Design review of the part built by this model. Coordinates are the model's own, in mm. A direction names the side the tool comes from. Give positions to 0.01 mm unless a question says otherwise; leave off trailing zeros. Order: outer loops, then holes, each group sorted by start corner. A loop starts at its lowest first (then second) coordinate and runs counter-clockwise, first axis right, second up. Notation, with made-up numbers: (47.5, -34) -> (104.5, -34) arc R27 cw to (104.5, -13) -> close; hole circle Ø2 at (-26.75, 45). An arc over 180 degrees is marked (long way). Return JSON: item names as keys, results as strings.
```python
from build123d import *

# Parameters (mm, degrees)
SKETCH_1_W               = 20
SKETCH_1_H               = 200
SKETCH_1_W_2             = 80
EXTRUDE_1_DEPTH          = 3
SKETCH_3_W               = 200
SKETCH_3_H               = 3
REVOLVE_1_ANGLE          = 90
SKETCH_5_W               = 200
SKETCH_5_H               = 3
REVOLVE_2_ANGLE          = 90
SKETCH_7_R               = 28.5
EXTRUDE_4_DEPTH          = 55
SKETCH_7_6_R             = 28.5
CUT_EXTRUDE_1_DEPTH      = 47
SKETCH_9_R               = 1.65
CUT_EXTRUDE_2_DEPTH      = 47
SKETCH_10_R              = 1.65
CUT_EXTRUDE_3_DEPTH      = 47
EXTRUDE_5_DEPTH          = 55
SKETCH_11_3_R            = 28.5
CUT_EXTRUDE_4_DEPTH      = 47
SKETCH_14_R              = 1.65
CUT_EXTRUDE_5_DEPTH      = 47
SKETCH_15_W              = 60
SKETCH_15_H              = 86
EXTRUDE_6_DEPTH          = 3
SKETCH_17_W              = 5
SKETCH_17_H              = 10
SKETCH_17_R              = 1.65
EXTRUDE_7_DEPTH          = 5
SKETCH_18_W              = 5
SKETCH_18_H              = 10
SKETCH_18_R              = 1.65
EXTRUDE_8_DEPTH          = 5
CUT_EXTRUDE_6_DEPTH      = 11
SKETCH_20_W              = 5.5
SKETCH_20_H              = 8.5
CUT_EXTRUDE_7_DEPTH      = 108
CUT_EXTRUDE_7_DEPTH_BACK = 119


with BuildPart() as part:
    # Sketch 1 → Extrude 1 (new body)
    with BuildSketch(Plane(origin=(0, 0, 0), x_dir=(1, 0, 0), z_dir=(0, 1, 0))):
        with Locations((-50, 0)):
            Rectangle(SKETCH_1_W, SKETCH_1_H)
        Rectangle(SKETCH_1_W_2, SKETCH_1_H)
        with Locations((50, 0)):
            Rectangle(SKETCH_1_W, SKETCH_1_H)
    extrude(amount=EXTRUDE_1_DEPTH)

    # Sketch 3 → Revolve 1 (revolve)
    with BuildSketch(Plane(origin=(60, 0, 0), x_dir=(0, 0, -1), z_dir=(1, 0, 0))):
        with Locations((0, 1.5)):
            Rectangle(SKETCH_3_W, SKETCH_3_H)
    revolve(axis=Axis((60, 33, 100), (0, 0, 1)), revolution_arc=REVOLVE_1_ANGLE)

    # Sketch 5 → Revolve 2 (revolve)
    with BuildSketch(Plane.ZY.offset(60)):
        with Locations((0, 1.5)):
            Rectangle(SKETCH_5_W, SKETCH_5_H)
    revolve(axis=Axis((-60, 33, -100), (0, 0, -1)), revolution_arc=REVOLVE_2_ANGLE)

    # Sketch 7 → Extrude 4 (add)
    with BuildSketch(Plane.XY.offset(100)):
        with Locations((-40, 40)):
            Circle(SKETCH_7_R)
        with BuildLine():
            Line((-60, 3), (-20, 3))
            Line((-20, 3), (-20, 19.696059496))
            ThreePointArc((-20, 19.696059496), (-40, 11.5), (-60, 19.696059496))
            Line((-60, 19.696059496), (-60, 3))
        make_face()
        with Locations((40, 40)):
            Circle(SKETCH_7_R)
        with BuildLine():
            Line((60, 3), (60, 19.696059496))
            ThreePointArc((60, 19.696059496), (40, 11.5), (20, 19.696059496))
            Line((20, 19.696059496), (20, 3))
            Line((20, 3), (60, 3))
        make_face()
    extrude(amount=-EXTRUDE_4_DEPTH)

    # Sketch 7_6 → Cut-Extrude 1 (cut)
    with BuildSketch(Plane.XY.offset(100)):
        with Locations((40, 40)):
            Circle(SKETCH_7_6_R)
        with Locations((-40, 40)):
            Circle(SKETCH_7_6_R)
    extrude(amount=-CUT_EXTRUDE_1_DEPTH, mode=Mode.SUBTRACT)

    # Sketch 9 → Cut-Extrude 2 (cut)
    with BuildSketch(Plane(origin=(0, 0, 45), x_dir=(-1, 0, 0), z_dir=(0, 0, -1))):
        with Locations((-53.435028843, 53.435028843)):
            Circle(SKETCH_9_R)
        with Locations((-26.564971157, 53.435028843)):
            Circle(SKETCH_9_R)
        with Locations((-26.564971157, 26.564971157)):
            Circle(SKETCH_9_R)
        with Locations((-53.435028843, 26.564971157)):
            Circle(SKETCH_9_R)
    extrude(amount=-CUT_EXTRUDE_2_DEPTH, mode=Mode.SUBTRACT)

    # Sketch 10 → Cut-Extrude 3 (cut)
    with BuildSketch(Plane(origin=(0, 0, 45), x_dir=(-1, 0, 0), z_dir=(0, 0, -1))):
        with Locations((26.564971157, 53.435028843)):
            Circle(SKETCH_10_R)
        with Locations((53.435028843, 53.435028843)):
            Circle(SKETCH_10_R)
        with Locations((53.435028843, 26.564971157)):
            Circle(SKETCH_10_R)
        with Locations((26.564971157, 26.564971157)):
            Circle(SKETCH_10_R)
    extrude(amount=-CUT_EXTRUDE_3_DEPTH, mode=Mode.SUBTRACT)

    # Sketch 11 → Extrude 5 (add)
    with BuildSketch(Plane(origin=(0, 0, -100), x_dir=(-1, 0, 0), z_dir=(0, 0, -1))):
        with BuildLine():
            Line((-20, 3), (-20, 19.696059496))
            ThreePointArc((-20, 19.696059496), (-40, 68.5), (-60, 19.696059496))
            Line((-60, 19.696059496), (-60, 3))
            Line((-60, 3), (-20, 3))
        make_face()
        with BuildLine():
            Line((20, 19.696059496), (20, 3))
            Line((20, 3), (60, 3))
            Line((60, 3), (60, 19.696059496))
            ThreePointArc((60, 19.696059496), (40, 68.5), (20, 19.696059496))
        make_face()
    extrude(amount=-EXTRUDE_5_DEPTH)

    # Sketch 11_3 → Cut-Extrude 4 (cut)
    with BuildSketch(Plane(origin=(0, 0, -100), x_dir=(-1, 0, 0), z_dir=(0, 0, -1))):
        with Locations((-40, 40)):
            Circle(SKETCH_11_3_R)
        with Locations((40, 40)):
            Circle(SKETCH_11_3_R)
    extrude(amount=-CUT_EXTRUDE_4_DEPTH, mode=Mode.SUBTRACT)

    # Sketch 14 → Cut-Extrude 5 (cut)
    with BuildSketch(Plane(origin=(0, 0, -53), x_dir=(-1, 0, 0), z_dir=(0, 0, -1))):
        with Locations((-26.564971157, 53.435028843)):
            Circle(SKETCH_14_R)
        with Locations((26.564971157, 53.435028843)):
            Circle(SKETCH_14_R)
        with Locations((-26.564971157, 26.564971157)):
            Circle(SKETCH_14_R)
        with Locations((-53.435028843, 26.564971157)):
            Circle(SKETCH_14_R)
        with Locations((-53.435028843, 53.435028843)):
            Circle(SKETCH_14_R)
        with Locations((53.435028843, 53.435028843)):
            Circle(SKETCH_14_R)
        with Locations((53.435028843, 26.564971157)):
            Circle(SKETCH_14_R)
        with Locations((26.564971157, 26.564971157)):
            Circle(SKETCH_14_R)
    extrude(amount=-CUT_EXTRUDE_5_DEPTH, mode=Mode.SUBTRACT)

    # Sketch 15 → Extrude 6 (add)
    with BuildSketch(Plane(origin=(0, 3, 0), x_dir=(1, 0, 0), z_dir=(0, 1, 0))):
        Rectangle(SKETCH_15_W, SKETCH_15_H)
    extrude(amount=EXTRUDE_6_DEPTH)

    # Sketch 17 → Extrude 7 (add)
    with BuildSketch(Plane.XY.offset(100)):
        with Locations((-10, 5)):
            Rectangle(SKETCH_17_W, SKETCH_17_H)
        with Locations((-10, 7)):
            Circle(SKETCH_17_R, mode=Mode.SUBTRACT)
        with Locations((10, 5)):
            Rectangle(SKETCH_17_W, SKETCH_17_H)
        with Locations((10, 7)):
            Circle(SKETCH_17_R, mode=Mode.SUBTRACT)
    extrude(amount=-EXTRUDE_7_DEPTH)

    # Sketch 18 → Extrude 8 (add)
    with BuildSketch(Plane(origin=(0, 0, -100), x_dir=(-1, 0, 0), z_dir=(0, 0, -1))):
        with Locations((-10, 5)):
            Rectangle(SKETCH_18_W, SKETCH_18_H)
        with Locations(Location((-10, 7, 0), (0, 0, 180))):
            Circle(SKETCH_18_R, mode=Mode.SUBTRACT)
        with Locations((10, 5)):
            Rectangle(SKETCH_18_W, SKETCH_18_H)
        with Locations(Location((10, 7, 0), (0, 0, 180))):
            Circle(SKETCH_18_R, mode=Mode.SUBTRACT)
    extrude(amount=-EXTRUDE_8_DEPTH)

    # Sketch 19 → Cut-Extrude 6 (cut)
    with BuildSketch(Plane(origin=(0, 3, 0), x_dir=(1, 0, 0), z_dir=(0, 1, 0))):
        with BuildLine():
            Line((-53, -25), (-53, 25))
            ThreePointArc((-53, 25), (-45, 33), (-37, 25))
            Line((-37, 25), (-37, -25))
            ThreePointArc((-37, -25), (-45, -33), (-53, -25))
        make_face()
        with BuildLine():
            Line((37, -25), (37, 25))
            ThreePointArc((37, 25), (45, 33), (53, 25))
            Line((53, 25), (53, -25))
            ThreePointArc((53, -25), (45, -33), (37, -25))
        make_face()
    extrude(amount=-CUT_EXTRUDE_6_DEPTH, mode=Mode.SUBTRACT)

    # Sketch 20 → Cut-Extrude 7 (cut, two sides)
    with BuildSketch(Plane(origin=(0, 0, 0), x_dir=(0, 0, -1), z_dir=(1, 0, 0))) as cut_extrude_7_sk:
        with Locations((-95.25, 18.75)):
            Rectangle(SKETCH_20_W, SKETCH_20_H)
        with Locations((95.25, 18.75)):
            Rectangle(SKETCH_20_W, SKETCH_20_H)
    extrude(amount=CUT_EXTRUDE_7_DEPTH, mode=Mode.SUBTRACT)
    extrude(cut_extrude_7_sk.sketch, amount=-CUT_EXTRUDE_7_DEPTH_BACK, mode=Mode.SUBTRACT)


solid = part.part
```
Item 1: Wall thickness on L1, parallel to Y at x = 10, z = -97.75; L2, parallel to Z at x = 20, y = 58.5; L3, parallel to X at y = 19, z = 79.5: over which ranges is each line inside the solid? List them lowest first. Write a range as [from, to].
Result set:
{"L1": "y = [0, 5.35], [8.65, 10]", "L2": "z = [-53, -45], [45, 53]", "L3": "x = [-89.88, -86.53], [-60, -59.27], [-20.73, -20], [20, 20.73], [59.27, 60], [86.53, 89.88]"}
Item 2: Mouldability with a two-part tool opening along Z and no side actions: class faces 1 (the face through (10, 10, -98)), 2 (the face through (-40, 40, 53)), 3 (the face through (-45, 2, -33)) as released by +Z, released by -Z, zero draft, split by the parting line, or undercut.
Result set:
{"face 1": "zero draft", "face 2": "released by +Z", "face 3": "undercut"}
Item 3: Add section A-A (y = 40). Give the boundary of the cut face in (x, z).
Result set:
{"outline": "(-68.5, -53) -> (-11.5, -53) -> (-11.5, -45) -> (-68.5, -45) -> close; (-68.5, 45) -> (-11.5, 45) -> (-11.5, 53) -> (-68.5, 53) -> close; (11.5, -53) -> (68.5, -53) -> (68.5, -45) -> (11.5, -45) -> close; (11.5, 45) -> (68.5, 45) -> (68.5, 53) -> (11.5, 53) -> close"}
Item 4: Add section C-C (x = -45). Give the boundary of the cut face in (y, z).
Result set:
{"outline": "(0, -100) -> (11.94, -100) -> (11.94, -53) -> (68.06, -53) -> (68.06, -45) -> (3, -45) -> (3, -33) -> (0, -33) -> close; (0, 33) -> (3, 33) -> (3, 45) -> (68.06, 45) -> (68.06, 53) -> (11.94, 53) -> (11.94, 100) -> (0, 100) -> close"}
Item 5: Machinability: for faces 4 (the face through (-58, 16, 98)), 5 (the face through (-39.7, 11.5, -76.8)), 6 (the face through (-10, 10, -98)), 7 (the face through (87, 19, 92.5)), which of the approach directions +Z, -Z, +X, -X, +Y, -Y give a long, thin tool a straight path to every point of the face, cutting with its end or side? Answer none if there is none.
Result set:
{"face 4": "+X, -X, +Y", "face 5": "-Z, +Y", "face 6": "+Z, -Z, +Y", "face 7": "+X, -X"}
Item 6: Add section B-B (z = -22.5). Give the boundary of the cut face in (x, y), plus the area to 3 significant figures.
Result set:
{"outline": "(-93, 33) arc R33 ccw to (-60, 0) -> (-53, 0) -> (-53, 3) -> (-60, 3) arc R30 cw to (-90, 33) -> close; (-37, 0) -> (37, 0) -> (37, 3) -> (30, 3) -> (30, 6) -> (-30, 6) -> (-30, 3) -> (-37, 3) -> close; (53, 0) -> (60, 0) arc R33 ccw to (93, 33) -> (90, 33) arc R30 cw to (60, 3) -> (53, 3) -> close", "area": "741 mm^2"}
Item 7: For pin 1 (3 mm diameter, centred on x = -85, z = 95.5, fed in from +Y); pin 2 (13.5 mm diameter, centred on y = 9, z = 80.5, fed in from -X); pin 3 (18.5 mm diameter, centred on y = 10.5, z = -76.5, fed in from -X), all flat-tipped, find the tip position at first contact; note any pin that passes through.
Result set:
{"pin 1": "stops at y = 14.5", "pin 2": "stops at x = -88.13", "pin 3": "stops at x = -90.22"}
Item 8: Add section D-D (x = 40). Give the boundary of the cut face in (y, z) (3 decimals).
Result set:
{"outline": "(0, -100) -> (11.5, -100) -> (11.5, -53) -> (68.5, -53) -> (68.5, -45) -> (3, -45) -> (3, -31.245) -> (0, -31.245) -> close; (0, 31.245) -> (3, 31.245) -> (3, 45) -> (68.5, 45) -> (68.5, 53) -> (11.5, 53) -> (11.5, 100) -> (0, 100) -> close"}
